Check sheet for the modelled part. Datum: model origin and axes. Units: mm. Face numbers are marked on the shaded views. A direction names the side the tool comes from. Give positions to 0.01 mm unless a question says otherwise; leave off trailing zeros. Order: outer loops, then holes, each group sorted by start corner. A loop starts at its lowest first (then second) coordinate and runs counter-clockwise, first axis right, second up.
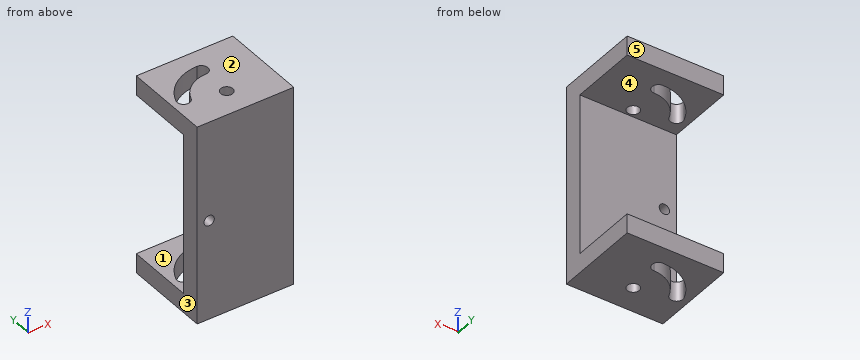
Autodesk Inventor part; units mm, degrees
ref_plane "YZ Plane" through (0, 0, 0) normal (1, 0, 0) x (0, 1, 0)
ref_plane "XZ Plane" through (0, 0, 0) normal (0, 1, 0) x (-1, 0, 0)
ref_plane "XY Plane" through (0, 0, 0) normal (0, 0, 1) x (1, 0, 0)
sketch "Sketch1" plane through (0, 0, 0) normal (0, 1, 0) x (-1, 0, 0)
  line L0 (0, 0) -> (19.05, 0)
  line L1 (19.05, 0) -> (19.05, -31.75)
  line L2 (19.05, -31.75) -> (0, -31.75)
  line L3 (0, -31.75) -> (0, 0)
  line L4 (19.05, 0) -> (19.05, 3.81)
  line L5 (19.05, 3.81) -> (0, 3.81)
  line L6 (0, 3.81) -> (0, 0)
  line L7 (19.05, -31.75) -> (19.05, -35.56)
  line L8 (19.05, -35.56) -> (0, -35.56)
  line L9 (0, -35.56) -> (0, -31.75)
  dimension "d0" = 19.05
  dimension "d1" = 31.75
  dimension "d4" = 3.81
  dimension "d5" = 3.81
extrude "Extrusion2" add sketch "Sketch1" along normal blind 9.525
sketch "Sketch3" plane through (0, 9.525, 0) normal (0, 1, 0) x (1, 0, 0)
  line L0 (0, 0) -> (-19.05, 0)
  line L1 (-19.05, 31.75) -> (0, 31.75)
  line L2 (0, 0) -> (0, 31.75)
  line L3 (-19.05, 31.75) -> (-19.05, 0)
  point P0 (-19.05, 35.56)
extrude "Extrusion3" cut sketch "Sketch3" against normal blind 5.715
sketch "Sketch4" plane through (0, 9.525, 0) normal (0, 1, 0) x (1, 0, 0)
  line L0 (-18.8776, 0) -> (0, 0)
  line L1 (0, 0) -> (0, -3.81)
  line L2 (0, -3.81) -> (-18.8776, -3.81)
  line L3 (-19.05, 35.56) -> (0, 35.56)
  line L4 (0, 35.56) -> (0, 31.75)
  line L5 (0, 31.75) -> (-19.05, 31.75)
  line L6 (-19.05, 31.75) -> (-19.05, 35.56)
  line L7 (-18.8776, 0) -> (-19.05, 0)
  line L8 (0, 0) -> (-19.05, 0)
  line L9 (-19.05, 0) -> (-19.05, -3.81)
  line L10 (-18.8776, -3.81) -> (-19.05, -3.81)
  line L11 (-19.05, -3.81) -> (0, -3.81)
extrude "Extrusion4" add sketch "Sketch4" along normal blind 7.62
sketch "Sketch5" plane through (0, 3.81, 0) normal (0, 1, 0) x (1, 0, 0)
  line L0 (-19.0656, 0) -> (0, 0)
  line L1 (0, 0) -> (0, 31.75)
  line L2 (0, 31.75) -> (-19.0656, 31.75)
  line L3 (-19.0656, 31.75) -> (-19.0656, 0)
  line L4 (0, 0) -> (-19.05, 0)
  line L5 (-19.05, 31.75) -> (0, 31.75)
  line L6 (-9.525, 0) -> (22.3112, 0) construction
  line L7 (-9.525, 31.75) -> (-9.525, 0)
  line L8 (-9.525, 0) -> (-9.525, 15.875)
  line L9 (-9.525, 15.875) -> (-9.525, 31.75)
  circle A0 centre (-16.6804, 15.875) radius 1.016
  point P0 (-18.8776, 0)
  dimension "d43" = 2.032
extrude "Extrusion5" cut sketch "Sketch5" against normal blind 3.81 contours A0
sketch "Sketch7" plane through (0, 0, -35.56) normal (0, 0, -1) x (-1, 0, 0)
  line L0 (19.05, 3.81) -> (0, 3.81)
  line L1 (0, 3.81) -> (0, 17.145)
  line L2 (0, 17.145) -> (19.05, 17.145)
  line L3 (19.05, 17.145) -> (19.05, 3.81)
  line L4 (19.05, 17.145) -> (0, 17.145)
  line L5 (19.05, 3.81) -> (0, 3.81)
  line L6 (0, 17.145) -> (0, 3.81)
  circle A0 centre (9.525, 12.3825) radius 1.016
  point P0 (0, 0)
  dimension "d42" = 2.032
extrude "Extrusion7" cut sketch "Sketch7" against normal blind 39.37 contours A0
sketch "Sketch13" plane through (-19.05, 0, 3.81) normal (0, 0, 1) x (1, 0, 0)
  arc A0 (9.5897, 13.6509) -> (9.4386, 13.6496) centre (9.525, 12.3825) ccw
  arc A1 (9.5359, 11.1125) -> (3.682, 6.9762) centre (9.5897, 4.826) ccw
  arc A2 (9.5897, 13.6509) -> (1.297, 7.8443) centre (9.5897, 4.826) ccw
  line L0 (9.5897, 4.826) -> (18.4145, 4.826) construction
  line L1 (9.5897, 4.826) -> (18.4145, 4.826) construction
  arc A3 (1.297, 7.8443) -> (3.682, 6.9762) centre (2.4895, 7.4102) ccw
  line L2 (9.5897, 4.826) -> (11.1137, 4.826) construction
  line L3 (9.5897, 6.5604) -> (9.5897, 5.3539)
  circle A4 centre (9.5897, 5.3539) radius 1.2065
  arc A5 (9.5359, 11.1125) -> (9.4386, 13.6496) centre (9.525, 12.3825) ccw
  point P0 (19.05, 0)
  point P1 (9.5897, 3.81)
extrude "Extrusion14" cut sketch "Sketch13" against normal blind 76.2
sketch "Sketch21" plane through (0, 0, 0) normal (0, -1, 0) x (1, 0, 0)
  point P0 (0, 0)
properties part number "landing-gear-ublock" material "ABS Plastic"
1) Section check C-C, the plane x = -11.25. Record the cut outline in (y, z) (3 decimals).
Recorded:
outline: (0, -35.56) - (10.853, -35.56) - (10.853, -31.75) - (3.81, -31.75) - (3.81, 0) - (10.853, 0) - (10.853, 3.81) - (0, 3.81) - close; (13.468, -35.56) - (17.145, -35.56) - (17.145, -31.75) - (13.468, -31.75) - close; (13.468, 0) - (17.145, 0) - (17.145, 3.81) - (13.468, 3.81) - close
2) Section check D-D, the plane y = 13. Record the cut outline in (x, z), then the cut area to 3 significant figures.
Recorded:
outline: (-19.05, -35.56) - (-12.79, -35.56) - (-12.79, -31.75) - (-19.05, -31.75) - close; (-19.05, 0) - (-12.79, 0) - (-12.79, 3.81) - (-19.05, 3.81) - close; (-8.42, -35.56) - (0, -35.56) - (0, -31.75) - (-8.42, -31.75) - close; (-8.42, 0) - (0, 0) - (0, 3.81) - (-8.42, 3.81) - close
area: 112 mm2
3) Section check A-A, the plane y = 16.25. Record the cut outline in (x, z), then the cut area to 3 significant figures.
Recorded:
outline: (-19.05, -35.56) - (0, -35.56) - (0, -31.75) - (-19.05, -31.75) - close; (-19.05, 0) - (0, 0) - (0, 3.81) - (-19.05, 3.81) - close
area: 145 mm2
4) Set-up check for the marked faces 4 and 5: record each of +Z, -Z, +X, -X, +Y, -Y from which the full face is reachable in a straight line by a thin tool's end or side.
Recorded:
face 4: +X, -X, +Y
face 5: +Z, -Z, +X, -X, +Y
5) Material ranges on L1, parallel to Z at x = -15, y = 13.25; L2, parallel to Y at x = -6.75, z = -20; L3, parallel to Y at x = -13.25, z = 2 (3 decimals), recorded low to high.
Recorded:
L1: z = -35.56 to -31.75, 0 to 3.81
L2: y = 0 to 3.81
L3: y = 0 to 9.842, 12.796 to 17.145
6) Section check B-B, the plane x = -16.25. Record the cut outline in (y, z) (3 decimals), then the cut area to 3 significant figures.
Recorded:
outline: (0, -35.56) - (6.18, -35.56) - (6.18, -31.75) - (3.81, -31.75) - (3.81, -16.795) - (0, -16.795) - close; (0, -14.955) - (3.81, -14.955) - (3.81, 0) - (6.18, 0) - (6.18, 3.81) - (0, 3.81) - close; (10.463, -35.56) - (17.145, -35.56) - (17.145, -31.75) - (10.463, -31.75) - close; (10.463, 0) - (17.145, 0) - (17.145, 3.81) - (10.463, 3.81) - close
area: 212 mm2
7) Draft check along Z on the marked faces 1, 2 and 3. Enter one of: +Z half, -Z half, draft (parallel to the pull), parting line (faces both ways), or undercut.
Recorded:
face 1: undercut
face 2: +Z half
face 3: draft
